Could you check a few things on this model? Use its own coordinates, in mm. Face numbers are marked on the shaded views. Give positions to 0.01 mm unless a question says otherwise; leave off trailing zeros. Order: outer loops, then holes, each group sorted by start corner. A loop starts at its lowest first (then second) coordinate and runs counter-clockwise, first axis right, second up. Notation, with made-up numbers: (79, 71) -> (115, 71) arc R29 ccw to (115, 110) -> close; hole circle Ø7 at (8, 80). An arc over 180 degrees is marked (long way). One line per item, written item: value.
```python
from build123d import *

# Parameters (mm, degrees)
F2_R     = 60.1927898824
F3_DEPTH = 1270
F4_R     = 5.08


with BuildPart() as f1:
    # F0 (on Front) → F1 (revolve)
    with BuildSketch(Plane.XZ):
        Polygon((37.8701165318, 56.4049184322), (-37.3361222446, 56.4049184322), (-37.3361222446, -67.5895376156), (-30.1177501678, -67.5895376156), (-30.1177501678, -60.6174655259), (-23.6104177256, -67.5895376156), (-12.9269050552, -60.6174655259), (-8.2385898663, -67.5895376156), (19.8104574267, -67.5895376156), (32.1801453829, -57.270154357), (32.1801453829, -67.5895376156), (37.8701165318, -67.5895376156), align=None)
    revolve(axis=Axis((0.2669971436, 0, 56.4049184322), (1, 0, 0)))

    # F2 (on Right) → F3 (cut, symmetric)
    with BuildSketch(Plane.YZ):
        with Locations((0, 60.1927898824)):
            Circle(F2_R)
    extrude(amount=F3_DEPTH, both=True, mode=Mode.SUBTRACT)

    # F4
    f4_edges = [f1.edges().sort_by_distance(p)[0] for p in [
        (37.870117, 0, 180.399374),
        (-37.336122, 0, 180.399374),
    ]]
    fillet(f4_edges, radius=F4_R)


solid = f1.part
```
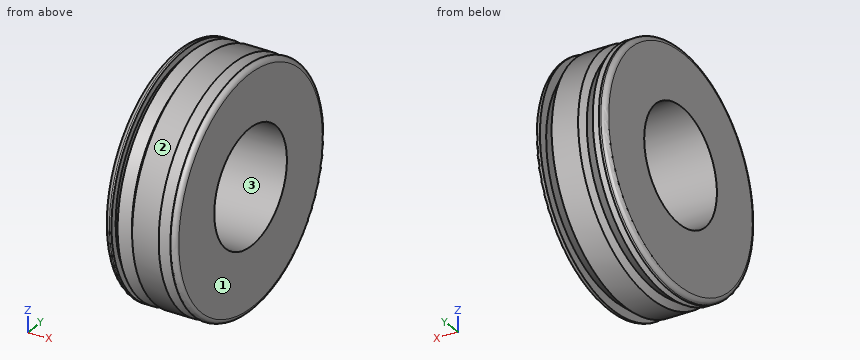
1) For P1, Ø12, axis at x = -18, z = 118, coming from the -Y side; P2, Ø12, axis at x = 22, y = 84.5, coming from the +Z side; P3, Ø12, axis at x = 15.5, y = -33, coming from the +Z side, each with a flat end and sliding along its axis, tell me the tip position at first contact or that it passes through.
Answer below:
P1: stops at y = -109
P2: stops at z = 152.05
P3: stops at z = 177.42
2) Suppose I cut it at A-A, the plane y = 0. Write out the boundary of the cut face in (x, z), then the cut area to 3 significant figures.
Answer below:
outline: (-37.34, -62.51) arc R5.08 ccw to (-32.26, -67.59) -> (-30.12, -67.59) -> (-30.12, -60.62) -> (-23.61, -67.59) -> (-12.93, -60.62) -> (-8.24, -67.59) -> (19.81, -67.59) -> (32.18, -57.27) -> (32.18, -67.59) -> (32.79, -67.59) arc R5.08 ccw to (37.87, -62.51) -> (37.87, 0) -> (-37.34, 0) -> close; (-37.34, 120.39) -> (37.87, 120.39) -> (37.87, 175.32) arc R5.08 ccw to (32.79, 180.4) -> (32.18, 180.4) -> (32.18, 170.08) -> (19.81, 180.4) -> (-8.24, 180.4) -> (-12.93, 173.43) -> (-23.61, 180.4) -> (-30.12, 173.43) -> (-30.12, 180.4) -> (-32.26, 180.4) arc R5.08 ccw to (-37.34, 175.32) -> close
area: 9,290 mm2
3) Suppose I cut it at B-B, the plane x = -19. Write out the boundary of the cut face in (y, z), then the cut area to 3 significant figures.
Answer below:
outline: circle Ø241.97 at (0, 56.4); hole circle Ø120.39 at (0, 60.19)
area: 34,600 mm2
4) We'd pull the mould along Z, two halves only. Please class the marked faces 1, 2 and 3: +Z half, -Z half, draft (parallel to the pull), parting line (faces both ways), or undercut.
Answer below:
face 1: draft
face 2: parting line
face 3: undercut
5) If I drill on line 1 along X through (y, z) = (50.5, -50); line 2 along X through (y, z) = (60.5, 162.5); line 3 along Y through (x, z) = (8, 108), over which ranges is the centre line in solid material (lowest first)?
Answer below:
line 1: x = -37.34 to -30.12, -29.41 to -14.09, -12.42 to 27.26, 32.18 to 37.87
line 2: x = -36.19 to -30.12, -25.35 to -20.76, -9.49 to 22.04, 32.18 to 36.72
line 3: y = -112.75 to -36.57, 36.57 to 112.75
